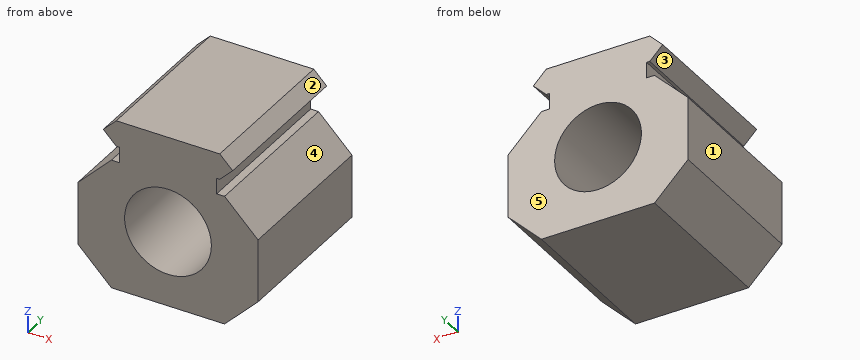
```python
from build123d import *

# Parameters (mm, degrees)
F1_DEPTH    = 25.4
F3_D        = 13.97
F3_DEPTH    = 25.4
F3_TIP      = 4.1970114239
F4_T1_DEPTH = 37.157734621


# Not quite as in the source:
# - a fillet or chamfer that OpenCascade refuses, or shapes differently, is made with other operations: its cross-section is extruded or revolved along the edge and cut away or added


with BuildPart() as f1:
    # F0 (on Front) → F1 (new body)
    with BuildSketch(Plane.XZ):
        Polygon((10.6172, 19.1102290041), (0, 19.1102290041), (0, -8.5316783412), (9.1059, -8.5316783412), (14.4940536726, -3.1435246685), (14.4940536726, 7.0164753315), (9.1059, 12.4046290041), (7.8359, 12.4046290041), (7.8359, 14.9446290041), (10.6172, 14.9446290041), align=None)
        Polygon((0, -8.5316783412), (0, 19.1102290041), (-10.6172, 19.1102290041), (-10.6172, 14.9446290041), (-7.8359, 14.9446290041), (-7.8359, 12.4046290041), (-9.1059, 12.4046290041), (-14.4940536726, 7.0164753315), (-14.4940536726, -3.1435246685), (-9.1059, -8.5316783412), align=None)
    extrude(amount=F1_DEPTH)

    # F3
    with Locations(Plane(origin=(0, 0, 0), x_dir=(-1, 0, 0), z_dir=(0, 1, 0))):
        with Locations((0, 3.620829666)):
            Hole(F3_D / 2, depth=F3_DEPTH)
            with Locations((0, 0, -(F3_DEPTH + F3_TIP / 2))):  # 118° drill point
                Cone(0, F3_D / 2, F3_TIP, mode=Mode.SUBTRACT)

    # F4: chamfer of 2.286 on 4 edges, made by hand

    # F4_s2 → F4_t1 (cut)
    with BuildSketch(Plane.XZ.offset(-5.8788673105)):
        Polygon((8.3312, 14.9446290041), (10.6172, 17.2306290041), (10.6172, 14.9446290041), align=None)
        Polygon((10.6172, 16.8242290041), (8.3312, 19.1102290041), (10.6172, 19.1102290041), align=None)
        Polygon((-8.3312, 19.1102290041), (-10.6172, 16.8242290041), (-10.6172, 19.1102290041), align=None)
        Polygon((-10.6172, 17.2306290041), (-8.3312, 14.9446290041), (-10.6172, 14.9446290041), align=None)
    extrude(amount=F4_T1_DEPTH, mode=Mode.SUBTRACT)


solid = f1.part
```
Verification items for the finished model (mm, model axes). Face numbers are marked on the shaded views. A direction names the side the tool comes from. Coordinates: 2 decimals unless noted, no trailing zeros. Write each loop counter-clockwise with the first axis right and the second up, starting at its lowest first coordinate (ties: lowest second). Pieces come first, ordered by that corner, then holes. Notation, with made-up numbers: (58, -17) - (111, -17) arc R9 cw to (111, -4) - close; hole circle Ø7 at (-4.75, -13.5). An arc over 180 degrees is marked (long way). Write item = value, one per line.
Q1. Cross-section at C-C (x = -10). Enter the section's corners in (y, z).
Answer:
outline = (-25.4, -7.64) - (0, -7.64) - (0, 11.51) - (-25.4, 11.51) - close; (-25.4, 16.61) - (0, 16.61) - (0, 17.44) - (-25.4, 17.44) - close
Q2. Cross-section at B-B (y = -20.5). Enter the section's corners in (x, z) (3 decimals).
Answer:
outline = (-14.494, -3.144) - (-9.106, -8.532) - (9.106, -8.532) - (14.494, -3.144) - (14.494, 7.016) - (9.106, 12.405) - (7.836, 12.405) - (7.836, 14.945) - (8.331, 14.945) - (10.414, 17.027) - (8.331, 19.11) - (-8.331, 19.11) - (-10.414, 17.027) - (-8.331, 14.945) - (-7.836, 14.945) - (-7.836, 12.405) - (-9.106, 12.405) - (-14.494, 7.016) - close; hole circle Ø13.97 at (0, 3.621)
Q3. Mould release check, pull along Z, two halves, no side actions. Record for the marked faces 1, 2 and 3: released by +Z, released by -Z, zero draft, split by the parting line, or undercut.
Answer:
face_1 = zero draft
face_2 = released by +Z
face_3 = undercut
Q4. Cross-section at A-A (x = 0). Enter the section's corners in (y, z).
Answer:
outline = (-25.4, -8.53) - (0, -8.53) - (0, -3.36) - (-25.4, -3.36) - close; (-25.4, 10.61) - (0, 10.61) - (0, 19.11) - (-25.4, 19.11) - close
Q5. Cross-section at D-D (z = 17.5). Enter the section's corners in (x, y).
Answer:
outline = (-9.94, -25.4) - (9.94, -25.4) - (9.94, 0) - (-9.94, 0) - close
Q6. Access from +Z, -Z, +X, -X, +Y, -Y to the whole of each face (thin tool, end or side, straight path). Record for the marked faces 4 and 5.
Answer:
face_4 = +X, +Y, -Y
face_5 = +Z, -Z, +X, -X, +Y
Q7. Material ranges on L1, parallel to Z at x = 0, y = -7.25; L2, parallel to X at y = -19.75, z = 0.5; L3, parallel to X at y = -2.75, z = 6.5, recorded low to high. Write a range as from..to.
Answer:
L1 = -8.53..-3.36, 10.61..19.11
L2 = -14.49..-6.25, 6.25..14.49
L3 = -14.49..-6.36, 6.36..14.49
Q8. Go/stop test with flat-tipped pins: pin 1 Ø12 at (x, y) = (9.5, -13) entering from +Z; pin 2 Ø3 at (y, z) = (-14, 13) entering from +X; pin 3 Ø2 at (y, z) = (-10, 13.5) entering from -X. Record where each tip stops, or that it passes through.
Answer:
pin_1 = 19.11
pin_2 = 10.01
pin_3 = -7.84
